Can you work these out from the model? Positions are in its coordinate system, mm. Face numbers are marked on the shaded views. A direction names the side the tool comes from. Coordinates: 2 decimals unless noted, no trailing zeros. Loops run counter-clockwise (first coordinate to the right, second up) from the corner with the lowest first, then second, coordinate; pieces in that order, holes last. Notation, with made-up numbers: M 34,85 L 61,85 A29 cw 61,110 Z; hole C 73,5.5 d9. An arc over 180 degrees is marked long. Return JSON: item names as keys, results as strings. Group by question number.
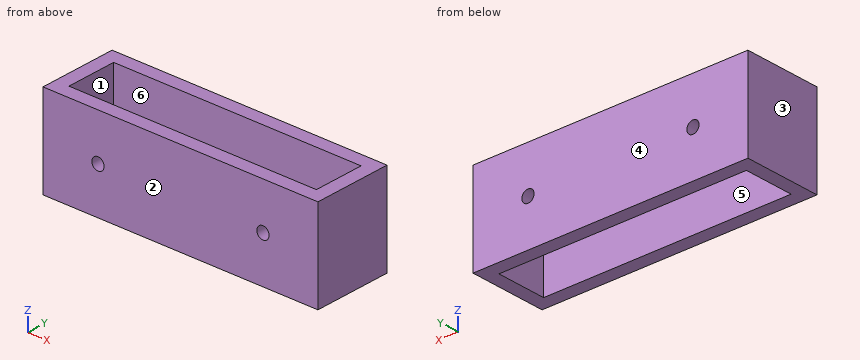
```python
from build123d import *

# Parameters (mm, degrees)
SKETCH1_W           = 150
SKETCH1_H           = 50
BOSS_EXTRUDE1_DEPTH = 7.5
SKETCH2_R           = 3.35
CUT_EXTRUDE1_DEPTH  = 7.5
SKETCH3_W           = 15
SKETCH3_H           = 50
BOSS_EXTRUDE2_DEPTH = 35
SKETCH6_W           = 50
SKETCH6_H           = 7.5
BOSS_EXTRUDE5_DEPTH = 120
SKETCH10_R          = 3.35
CUT_EXTRUDE4_DEPTH  = 7.5
SKETCH11_W          = 50
SKETCH11_H          = 27.5
CUT_EXTRUDE5_DEPTH  = 7.5
SKETCH12_W          = 50
SKETCH12_H          = 27.5
CUT_EXTRUDE6_DEPTH  = 7.5


with BuildPart() as part:
    # Sketch1 → Boss-Extrude1 (new body)
    with BuildSketch(Plane(origin=(0, 0, 0), x_dir=(1, 0, 0), z_dir=(0, 1, 0))):
        Rectangle(SKETCH1_W, SKETCH1_H)
    extrude(amount=BOSS_EXTRUDE1_DEPTH)

    # Sketch2 → Cut-Extrude1 (cut)
    with BuildSketch(Plane(origin=(0, 7.5, 0), x_dir=(1, 0, 0), z_dir=(0, 1, 0))):
        with Locations(Location((-45, 0, 0), (0, 0, 270))):
            Circle(SKETCH2_R)
        with Locations(Location((45, 0, 0), (0, 0, 270))):
            Circle(SKETCH2_R)
    extrude(amount=-CUT_EXTRUDE1_DEPTH, mode=Mode.SUBTRACT)

    # Sketch3 → Boss-Extrude2 (add)
    with BuildSketch(Plane.XZ):
        with Locations((-67.5, 0)):
            Rectangle(SKETCH3_W, SKETCH3_H)
        with Locations((67.5, 0)):
            Rectangle(SKETCH3_W, SKETCH3_H)
    extrude(amount=BOSS_EXTRUDE2_DEPTH)

    # Sketch6 → Boss-Extrude5 (add)
    with BuildSketch(Plane(origin=(-60, 0, 0), x_dir=(0, 0, -1), z_dir=(1, 0, 0))):
        with Locations((0, -31.25)):
            Rectangle(SKETCH6_W, SKETCH6_H)
    extrude(amount=BOSS_EXTRUDE5_DEPTH)

    # Sketch10 → Cut-Extrude4 (cut)
    with BuildSketch(Plane(origin=(0, -27.5, 0), x_dir=(1, 0, 0), z_dir=(0, 1, 0))):
        with Locations(Location((-45, 0, 0), (0, 0, 270))):
            Circle(SKETCH10_R)
        with Locations(Location((45, 0, 0), (0, 0, 270))):
            Circle(SKETCH10_R)
    extrude(amount=-CUT_EXTRUDE4_DEPTH, mode=Mode.SUBTRACT)

    # Sketch11 → Cut-Extrude5 (cut)
    with BuildSketch(Plane(origin=(-60, 0, 0), x_dir=(0, 0, -1), z_dir=(1, 0, 0))):
        with Locations((0, -13.75)):
            Rectangle(SKETCH11_W, SKETCH11_H)
    extrude(amount=-CUT_EXTRUDE5_DEPTH, mode=Mode.SUBTRACT)

    # Sketch12 → Cut-Extrude6 (cut)
    with BuildSketch(Plane.ZY.offset(-60)):
        with Locations((0, -13.75)):
            Rectangle(SKETCH12_W, SKETCH12_H)
    extrude(amount=-CUT_EXTRUDE6_DEPTH, mode=Mode.SUBTRACT)


solid = part.part
```
1) Suppose I cut it at A-A, the plane x = -17. List the corners of the cut face in (y, z) for me.
2) If we mould it in two halves opening along X, with no side actions, what happens to the marked faces 3, 4, 5 and 6? For each: +X half, -X half, draft (parallel to the pull), parting line (faces both ways), or undercut.
3) For pin 1 (4 mm diameter, centred on x = 45, z = 0, fed in from -Y), with a flat end and sliding along its axis, tell me the tip position at first contact or that it passes through.
4) If I drill on line 1 (X direction, y = 3, z = 0); line 2 (Y direction, x = 5, z = 16); line 3 (X direction, y = -18.5, z = 14), over which ranges is the centre line in solid material (lowest first)? Write a range as from..to.
5) For the marked faces 1 and 2, which set-ups out of +Z, -Z, +X, -X, +Y, -Y let a thin tool reach every point of the face, with its end or its side?
6) Suppose I cut it at D-D, the plane x = 45. List the corners of the cut face in (y, z) for me.
7) Suppose I cut it at C-C, the plane y = -13. List the corners of the cut face in (x, z) for me.
8) Suppose I cut it at B-B, the plane z = 0. List the corners of the cut face in (x, y) for me.
Returned:
{
 "1": {"outline": "M -35,-25 L -27.5,-25 L -27.5,25 L -35,25 Z; M 0,-25 L 7.5,-25 L 7.5,25 L 0,25 Z"},
 "2": {"face 3": "-X half", "face 4": "draft", "face 5": "undercut", "face 6": "undercut"},
 "3": {"pin 1": "passes through"},
 "4": {"line 1": "x = -75..-48.35, -41.65..41.65, 48.35..75", "line 2": "y = -35..-27.5, 0..7.5", "line 3": "x = -75..-67.5, 67.5..75"},
 "5": {"face 1": "+Z, -Z", "face 2": "+Z, -Z, +X, -X, -Y"},
 "6": {"outline": "M -35,-25 L -27.5,-25 L -27.5,-3.35 L -35,-3.35 Z; M -35,3.35 L -27.5,3.35 L -27.5,25 L -35,25 Z; M 0,-25 L 7.5,-25 L 7.5,-3.35 L 0,-3.35 Z; M 0,3.35 L 7.5,3.35 L 7.5,25 L 0,25 Z"},
 "7": {"outline": "M -75,-25 L -67.5,-25 L -67.5,25 L -75,25 Z; M 67.5,-25 L 75,-25 L 75,25 L 67.5,25 Z"},
 "8": {"outline": "M -75,-35 L -48.35,-35 L -48.35,-27.5 L -67.5,-27.5 L -67.5,0 L -48.35,0 L -48.35,7.5 L -75,7.5 Z; M -41.65,-35 L 41.65,-35 L 41.65,-27.5 L -41.65,-27.5 Z; M -41.65,0 L 41.65,0 L 41.65,7.5 L -41.65,7.5 Z; M 48.35,-35 L 75,-35 L 75,7.5 L 48.35,7.5 L 48.35,0 L 67.5,0 L 67.5,-27.5 L 48.35,-27.5 Z"}
}
